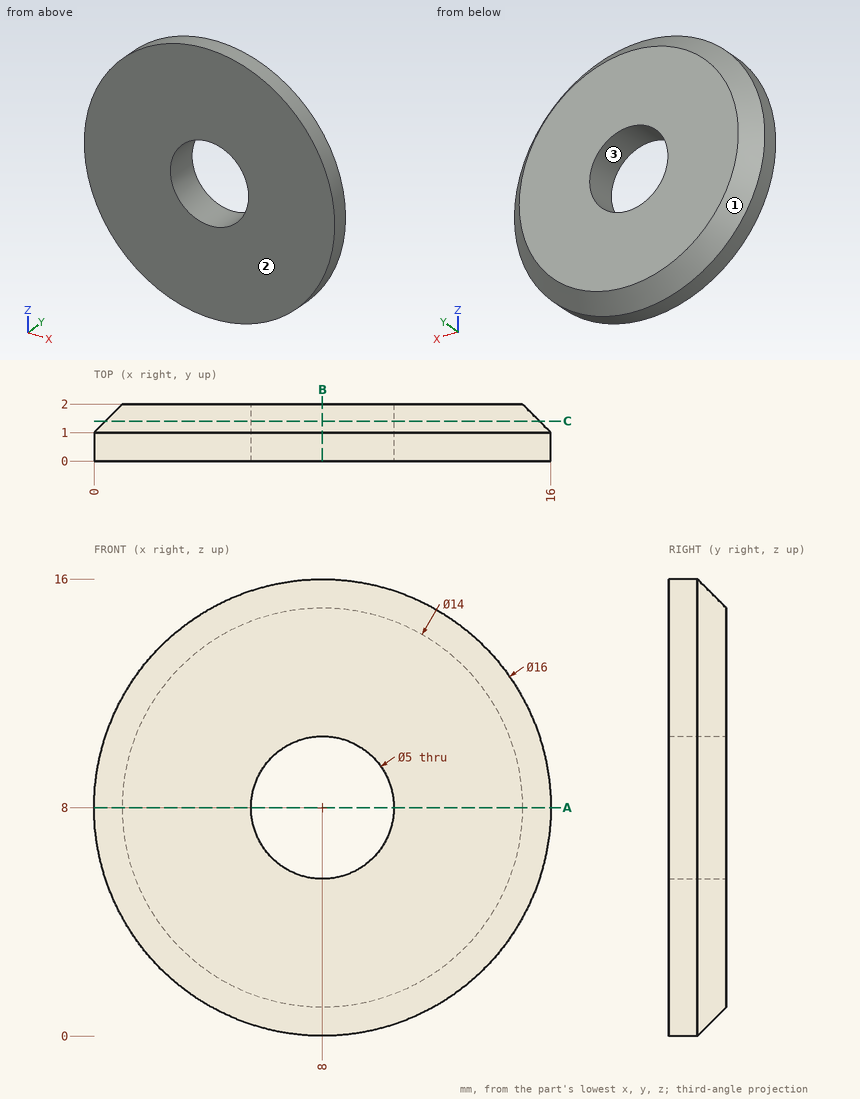
Input: dimensioned drawing with shaded views. Units: mm. Origin: part minimum x, y, z. Give positions to 0.01 mm unless a question says otherwise; leave off trailing zeros. Loops run counter-clockwise (first coordinate to the right, second up) from the corner with the lowest first, then second, coordinate; pieces in that order, holes last. Notation, with made-up numbers: (38.5, -8) -> (91.5, -8) arc R18 ccw to (91.5, 1) -> close; hole circle Ø11 at (31, 2.25). An arc over 180 degrees is marked (long way). Use a Markdown table: item, result.
Q1. Section query B-B, the plane x = 8. Return the cut outline in (y, z).
Entries:
| item | result |
|---|---|
| outline | (0, 0) -> (1, 0) -> (2, 1) -> (2, 5.5) -> (0, 5.5) -> close; (0, 10.5) -> (2, 10.5) -> (2, 15) -> (1, 16) -> (0, 16) -> close |
Q2. Ray query, probe 1 along X at (y, z) = (0.65, 8); probe 2 along X at (y, z) = (1.2, 8); probe 3 along Z at (x, y) = (8, 1.6). Return the intervals inside material, ascending. Write a range as from..to.
Entries:
| item | result |
|---|---|
| probe 1 | x = 0..5.5, 10.5..16 |
| probe 2 | x = 0.2..5.5, 10.5..15.8 |
| probe 3 | z = 0.6..5.5, 10.5..15.4 |
Q3. First-contact query: P1, Ø4.5, axis at x = 8, z = 8, coming from the -Y side. Flat tip, straight axial feed; report the tip coordinate or a pass-through.
Entries:
| item | result |
|---|---|
| P1 | passes through |
Q4. Section query A-A, the plane z = 8. Return the cut outline in (x, y), plus the area to 3 significant figures.
Entries:
| item | result |
|---|---|
| outline | (0, 0) -> (5.5, 0) -> (5.5, 2) -> (1, 2) -> (0, 1) -> close; (10.5, 0) -> (16, 0) -> (16, 1) -> (15, 2) -> (10.5, 2) -> close |
| area | 21.0 mm² |
Q5. Pull-direction query (Z, two-part tool) for the marked faces 1, 2 and 3; classes: pulls with the +Z half, pulls with the -Z half, needs draft (parallel to the pull), parting line crosses it, or undercut.
Entries:
| item | result |
|---|---|
| face 1 | parting line crosses it |
| face 2 | needs draft |
| face 3 | undercut |
Q6. Section query C-C, the plane y = 1.4. Return the cut outline in (x, z).
Entries:
| item | result |
|---|---|
| outline | circle Ø15.2 at (8, 8); hole circle Ø5 at (8, 8) |
